from build123d import *

# Parameters (mm, degrees)
EXTRUDE_1_DEPTH     = 10
CUT_EXTRUDE_1_REACH = 27.475
SKETCH_2_R          = 1.5
CUT_EXTRUDE_START   = -3
SKETCH_2_3_R        = 1.5
CUT_EXTRUDE_2_DEPTH = 2
CUT_EXTRUDE_3_REACH = 24.891
SKETCH_3_R          = 1.5


with BuildPart() as part:
    # 草图1 → 凸台-拉伸1 (new body)
    with BuildSketch(Plane.XY):
        Polygon((0, 0), (0, 15), (-5, 15), (-5, 5), (-18, 5), (-18, 0), align=None)
    extrude(amount=EXTRUDE_1_DEPTH)

    # 草图2 → 切除-拉伸1 (cut, up to next)
    with BuildSketch(Plane(origin=(0, 0, 0), x_dir=(0, 0, -1), z_dir=(1, 0, 0)), mode=Mode.PRIVATE) as cut_extrude_1_sk1:
        with Locations((-5, 10)):
            Circle(SKETCH_2_R)
    cut_extrude_1_tool1 = extrude(cut_extrude_1_sk1.sketch, amount=-CUT_EXTRUDE_1_REACH, mode=Mode.PRIVATE) & part.part
    add(cut_extrude_1_tool1.solids().sort_by_distance((0, 10, 5))[0], mode=Mode.SUBTRACT)

    # 草图2<3> → 切除-拉伸2 (cut)
    with BuildSketch(Plane(origin=(0, 0, 0), x_dir=(0, 0, -1), z_dir=(1, 0, 0)).offset(CUT_EXTRUDE_START)):
        Polygon((-5, 6.824573519), (-2.25, 8.41228676), (-2.25, 11.58771324), (-5, 13.175426481), (-7.75, 11.58771324), (-7.75, 8.41228676), align=None)
        with Locations((-5, 10)):
            Circle(SKETCH_2_3_R, mode=Mode.SUBTRACT)
    extrude(amount=-CUT_EXTRUDE_2_DEPTH, mode=Mode.SUBTRACT)

    # 草图3 → 切除-拉伸3 (cut, up to next)
    with BuildSketch(Plane(origin=(0, 5, 0), x_dir=(1, 0, 0), z_dir=(0, 1, 0)), mode=Mode.PRIVATE) as cut_extrude_3_sk1:
        with Locations(Location((-10, -5, 0), (0, 0, 180))):
            Circle(SKETCH_3_R)
    cut_extrude_3_tool1 = extrude(cut_extrude_3_sk1.sketch, amount=-CUT_EXTRUDE_3_REACH, mode=Mode.PRIVATE) & part.part
    add(cut_extrude_3_tool1.solids().sort_by_distance((-10, 5, 5))[0], mode=Mode.SUBTRACT)


solid = part.part
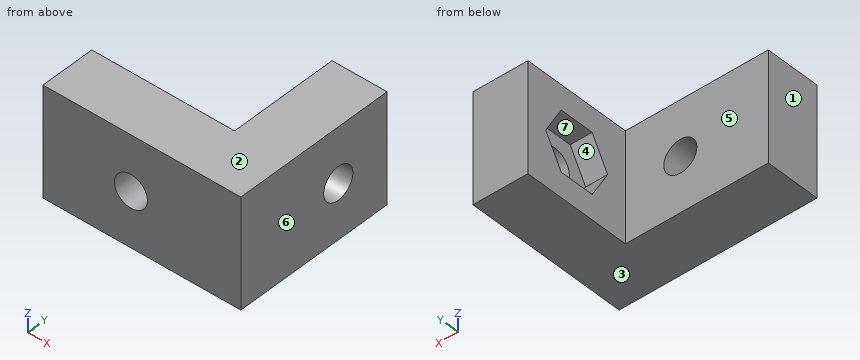
For this review, take the finished solid that the model builds, in its own axes (mm). Face numbers are marked on the shaded views. A direction names the side the tool comes from. Give positions to 0.01 mm unless a question says otherwise; leave off trailing zeros. Order: outer loops, then holes, each group sorted by start corner. A loop starts at its lowest first (then second) coordinate and runs counter-clockwise, first axis right, second up. Notation, with made-up numbers: M 76,22 L 122,22 A21 cw 122,51 Z; hole C 41,78.25 d1. An arc over 180 degrees is marked long. Answer in a Markdown table with one row per item. Add a question column.
(1) Consider section D-D on z = 8. State the section outline as (x, y) points.
(2) Consider section B-B on y = 10. State the section outline as (x, z) points, and give its area (3 significant figures).
(3) Wall thickness on probe 1 along Y at (x, z) = (-1.75, 5); probe 2 along Z at (x, y) = (-10, 3.5); probe 3 along Y at (x, z) = (-11.25, 2.5): over which ranges is each line inside the solid? List them lowest first. Write a range as [from, to].
(4) For pin 1 (1 mm diameter, centred on y = 3, z = 5, fed in from +X); pin 2 (2 mm diameter, centred on x = -9, z = 6.5, fed in from +Y); pin 3 (4.5 mm diameter, centred on y = 10, z = 6.5, fed in from -X); pin 4 (3.5 mm diameter, centred on y = 10, z = 5, fed in from -X), all flat-tipped, find the tip position at first contact; note any pin that passes through.
(5) Consider section A-A on x = -10. State the section outline as (y, z) points, and give its area (3 significant figures).
(6) For the marked faces 5, 6 and 7, list the 3-axis set-ups (+Z, -Z, +X, -X, +Y, -Y) from which the entire face can be reached by the end or side of a thin tool; tool diameter is ignored.
(7) Mouldability with a two-part tool opening along Z and no side actions: class the marked faces 1, 2, 3 and 4 as +Z half, -Z half, draft (parallel to the pull), parting line (faces both ways), or undercut.
(8) Consider section C-C on x = -4.25. State the section outline as (y, z) points, and give its area (3 significant figures).
Evaluation:
| question | item | result |
|---|---|---|
| 1 | outline | M -18,0 L 0,0 L 0,15 L -5,15 L -5,5 L -18,5 Z |
| 2 | outline | M -5,0 L 0,0 L 0,3.5 L -3,3.5 L -3,2.25 L -5,2.25 Z; M -5,7.75 L -3,7.75 L -3,6.5 L 0,6.5 L 0,10 L -5,10 Z |
| 2 | area | 30.0 mm^2 |
| 3 | probe 1 | y = [0, 8.5], [11.5, 15] |
| 3 | probe 2 | z = [0, 3.5], [6.5, 10] |
| 3 | probe 3 | y = [0, 5] |
| 4 | pin 1 | stops at x = 0 |
| 4 | pin 2 | stops at y = 5 |
| 4 | pin 3 | stops at x = -5 |
| 4 | pin 4 | stops at x = -3 |
| 5 | outline | M 0,0 L 5,0 L 5,3.5 L 0,3.5 Z; M 0,6.5 L 5,6.5 L 5,10 L 0,10 Z |
| 5 | area | 35.0 mm^2 |
| 6 | face 5 | +Z, -Z, -X, +Y |
| 6 | face 6 | +Z, -Z, +X, +Y, -Y |
| 6 | face 7 | -X |
| 7 | face 1 | draft |
| 7 | face 2 | +Z half |
| 7 | face 3 | -Z half |
| 7 | face 4 | undercut |
| 8 | outline | M 0,0 L 15,0 L 15,10 L 0,10 Z; hole M 6.82,5 L 8.41,2.25 L 11.59,2.25 L 13.18,5 L 11.59,7.75 L 8.41,7.75 Z |
| 8 | area | 124 mm^2 |
